The drawing under review shows one solid part. Ordinate dimensions are in mm from its lowest x, y, z. Coordinates: 2 decimals unless noted, no trailing zeros. Loops run counter-clockwise (first coordinate to the right, second up) from the corner with the lowest first, then second, coordinate; pieces in that order, holes last.
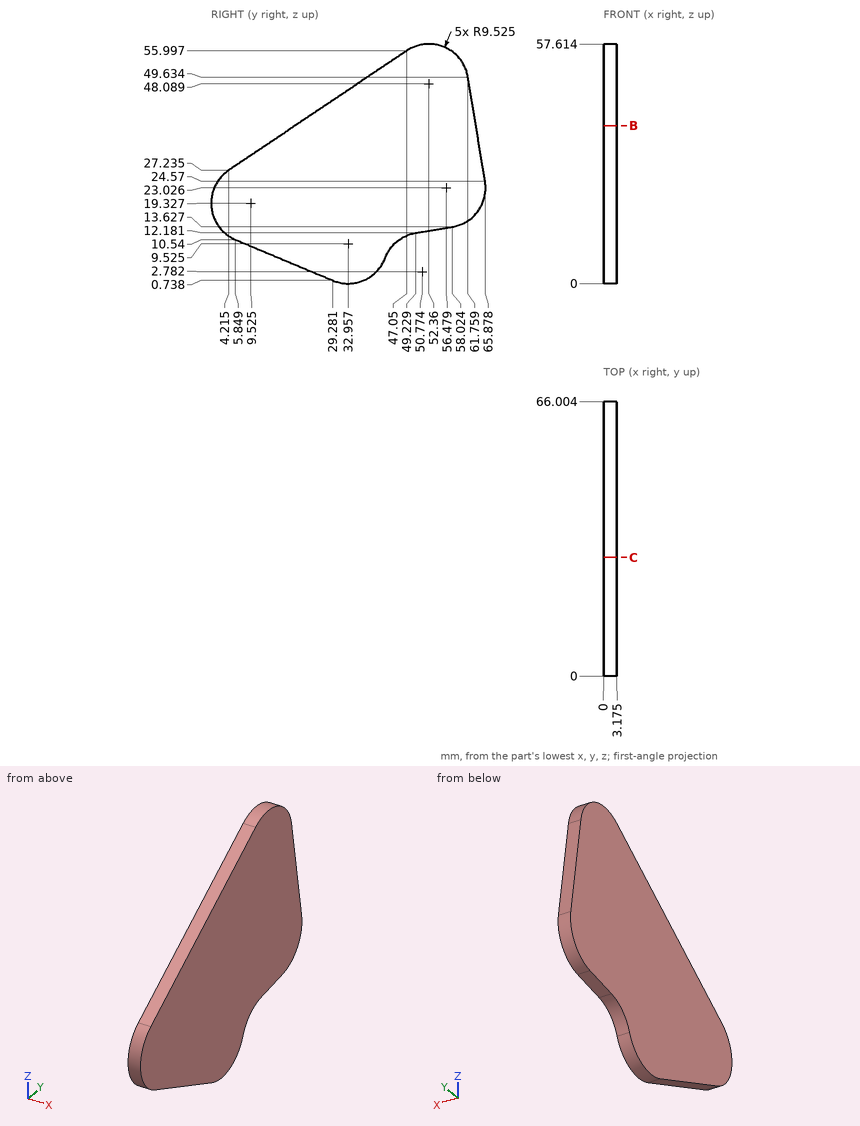
Q1. For line 1 (Z direction, x = 0.9, y = 7.5); line 2 (Z direction, x = 1.6, y = 40.5) (1 decimal); line 3 (Y direction, x = 2.95, z = 25.5) (1 decimal), list the stretches that pass through material, from the lowest coordinate up.
Q2. Take a section at B-B, the plane z = 38. Write out the cut boundary in (x, y) (1 decimal).
Q3. Take a section at C-C, the plane y = 28.5. Write out the cut boundary in (x, z) (1 decimal), then the cut area to 3 significant figures.
Entries:
1. line 1: z = 9.85 to 29.44
1. line 2: z = 3.7 to 51.6
1. line 3: y = 2.3 to 65.7
2. outline: (0, 20.2) - (3.2, 20.2) - (3.2, 63.7) - (0, 63.7) - close
3. outline: (0, 1.1) - (3.2, 1.1) - (3.2, 43.5) - (0, 43.5) - close
3. area: 135 mm2
